Build history of the part. All positions in model axes, mm. Face numbers are marked on the shaded views. A direction names the side the tool comes from. Give positions to 0.01 mm unless a question says otherwise; leave off trailing zeros. Order: outer loops, then holes, each group sorted by start corner. A loop starts at its lowest first (then second) coordinate and runs counter-clockwise, first axis right, second up. Notation, with made-up numbers: (15, 16.25) - (52, 16.25) arc R18 ccw to (52, 22.25) - close; hole circle Ø11 at (-13, 19). An arc over 180 degrees is marked (long way). Use a Markdown table: item, result.
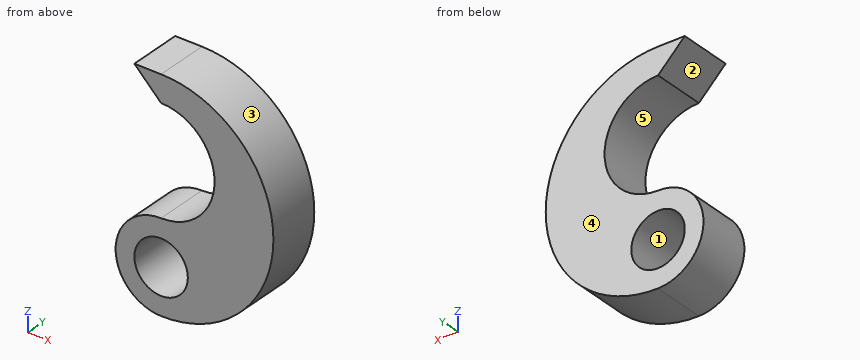
from build123d import *

# Parameters (mm, degrees)
F0_R     = 10
F1_DEPTH = 10


with BuildPart() as f1:
    # F0 (on Front) → F1 (new body, symmetric)
    with BuildSketch(Plane.XZ):
        with BuildLine():
            ThreePointArc((0, 17), (-17, 0), (0, -17))
            ThreePointArc((0, -17), (42, 25), (0, 67))
            Line((0, 67), (-10, 67))
            Line((-10, 67), (0, 57))
            ThreePointArc((0, 57), (20, 37), (0, 17))
        make_face()
        Circle(F0_R, mode=Mode.SUBTRACT)
    extrude(amount=F1_DEPTH, both=True)


solid = f1.part
1) Wall check: line 1 (Z direction, x = 6.5, y = 4.25); line 2 (Z direction, x = 4.5, y = 4.75); line 3 (X direction, y = 9.25, z = -9). Give the ranges that are in metal, low to high. Write a range as from..to.
Computed:
| item | result |
|---|---|
| line 1 | z = -16.49..-7.6, 7.6..18.09, 55.91..66.49 |
| line 2 | z = -16.76..-8.93, 8.93..17.51, 56.49..66.76 |
| line 3 | x = -14.42..-4.36, 4.36..24.66 |
2) Slice it at D-D (x = 6). Write the cut outline in (y, z).
Computed:
| item | result |
|---|---|
| outline | (-10, -16.57) - (10, -16.57) - (10, -8) - (-10, -8) - close; (-10, 8) - (10, 8) - (10, 17.92) - (-10, 17.92) - close; (-10, 56.08) - (10, 56.08) - (10, 66.57) - (-10, 66.57) - close |
3) Pin check, flat tips, straight feed: P1, Ø2, axis at y = 7, z = 2, coming from the +X side; P2, Ø8, axis at x = -2, y = -5.5, coming from the -Z side; P3, Ø16, axis at x = 0, z = 0, coming from the -Y side; P4, Ø6, axis at y = -6, z = 35.5, coming from the +X side. Stop position of each tip, or through.
Computed:
| item | result |
|---|---|
| P1 | stops at x = 35.78 |
| P2 | stops at z = -17 |
| P3 | passes through |
| P4 | stops at x = 41.32 |
4) Slice it at C-C (x = 13). Write the cut outline in (y, z), and give its area (3 significant figures).
Computed:
| item | result |
|---|---|
| outline | (-10, -14.94) - (10, -14.94) - (10, 21.8) - (-10, 21.8) - close; (-10, 52.2) - (10, 52.2) - (10, 64.94) - (-10, 64.94) - close |
| area | 990 mm² |
5) Tool access for the marked faces 1 and 2: list every direction of +Z, -Z, +X, -X, +Y, -Y with a clear straight run to the whole face (end or side of a thin tool).
Computed:
| item | result |
|---|---|
| face 1 | +Y, -Y |
| face 2 | -X, +Y, -Y |
6) Slice it at A-A (y = -7.25). Write the cut outline in (x, z), and give its area (3 significant figures).
Computed:
| item | result |
|---|---|
| outline | (-10, 67) - (0, 57) arc R20 cw to (0, 17) arc R17 ccw to (0, -17) arc R42 ccw to (0, 67) - close; hole circle Ø20 at (0, 0) |
| area | 2,330 mm² |
7) Two-plate mould, pull along Z, no slides. Class the marked faces 3, 4 and 5: +Z half, -Z half, draft (parallel to the pull), parting line (faces both ways), or undercut.
Computed:
| item | result |
|---|---|
| face 3 | parting line |
| face 4 | draft |
| face 5 | undercut |
8) Slice it at B-B (z = 0). Write the cut outline in (x, y), and give its area (3 significant figures).
Computed:
| item | result |
|---|---|
| outline | (-17, -10) - (-10, -10) - (-10, 10) - (-17, 10) - close; (10, -10) - (33.75, -10) - (33.75, 10) - (10, 10) - close |
| area | 615 mm² |
